Geometry: final body of the model. Coordinates: model frame, mm. A direction names the side the tool comes from. Give positions to 0.01 mm unless a question says otherwise; leave off trailing zeros. Loops run counter-clockwise (first coordinate to the right, second up) from the corner with the lowest first, then second, coordinate; pieces in that order, holes last. Notation, with made-up numbers: (46.25, 23) -> (93.25, 23) arc R23 cw to (93.25, 61) -> close; hole circle Ø6 at (49, -39.5). An arc over 180 degrees is marked (long way). One line per question, with ' | ' between items. Start each with the question number.
Item 1: Mould query, pull axis Y, two halves, no side actions, for faces 6 (the flat face through (0, 12, 11)), 7 (the flat face through (7, 25.725, 11)), 8 (the flat face through (15, -15, 11)). Classes: released by +Y, released by -Y, zero draft, split by the parting line, or undercut.
Item 2: Material intervals for line 1 along Y through (x, z) = (5.5, 11.25) (3 decimals); line 2 along X through (y, z) = (-7.5, 9.5) (3 decimals); line 3 along X through (y, z) = (14.5, 7), sorted ascending. Write a range as [from, to].
Item 3: Pin query (flat end, axial travel): P1, Ø1.5, axis at x = -49, z = 19, coming from the +Y side; P2, Ø6, axis at y = 1.5, z = 19.5, coming from the -X side; P3, Ø4, axis at x = -52, z = 13, coming from the -Y side; P4, Ø6.5, axis at y = -14.5, z = 8.5, coming from the +X side. Return the tip coordinate at first contact, or that it passes through.
Item 4: Section B-B on z = 12.25. Return loops of the section in (x, y) (3 decimals), then the cut area to 3 significant figures.
Item 5: Set-up query: faces 1 (the flat face through (-25, -20, 11)), 2 (the flat face through (7, 19, 17.725)), 3 (the flat face through (-49, -5, 11)), 4 (the flat face through (-51.9, -10, 21.2)), 5 (the flat face through (-11.7, -0.2, 22)). Return all of +Z, -Z, +X, -X, +Y, -Y with unobstructed straight access to the full face (end or side cutting, diameter ignored); none if empty.
Item 6: Section C-C on y = 8.5. Return loops of the section in (x, z), then the cut area to 3 significant figures.
Item 7: Section A-A on x = 1.5. Return loops of the section in (y, z) (3 decimals).
Item 8: Section D-D on x = -20.5. Return loops of the section in (y, z).
from build123d import *

# Parameters (mm, degrees)
PAD_DEPTH       = 22
SKETCH001_W     = 13.45
SKETCH001_H     = 13.45
POCKET_DEPTH    = 15
SKETCH002_W     = 13.45
SKETCH002_H     = 13.45
POCKET001_DEPTH = 15
CHAMFER_SIZE    = 10
POCKET002_DEPTH = 5
CHAMFER001_SIZE = 2


with BuildPart() as part:
    # Sketch → Pad (new body)
    with BuildSketch(Plane.XY):
        Polygon((0, 30), (0, 0), (-60, 0), (-60, -20), (20, -20), (20, 30), align=None)
    extrude(amount=PAD_DEPTH)

    # Sketch001 (on Face1 of Pad) → Pocket (cut)
    with BuildSketch(Plane(origin=(0, 0, 0), x_dir=(0, -1, 0), z_dir=(-1, 0, 0))):
        with Locations((-19, 11)):
            Rectangle(SKETCH001_W, SKETCH001_H)
    extrude(amount=-POCKET_DEPTH, mode=Mode.SUBTRACT)

    # Sketch002 (on Face12 of Pocket) → Pocket001 (cut)
    with BuildSketch(Plane.XZ.offset(20)):
        with Locations((-49, 11)):
            Rectangle(SKETCH002_W, SKETCH002_H)
    extrude(amount=-POCKET001_DEPTH, mode=Mode.SUBTRACT)

    # Chamfer
    chamfer_edges = [part.edges().sort_by_distance(p)[0] for p in [
        (20, -20, 11),
    ]]
    chamfer(chamfer_edges, length=CHAMFER_SIZE)

    # Sketch003 (on Face9 of Chamfer) → Pocket002 (cut)
    with BuildSketch(Plane.XY.offset(22)):
        Polygon((9.295837, 17.3), (10.704163, 17.3), (11.7, 18.295837), (11.7, 19.704163), (10.704163, 20.7), (9.295837, 20.7), (8.3, 19.704163), (8.3, 18.295837), align=None)
        Polygon((-47.3, -10.704163), (-47.3, -9.295837), (-48.295837, -8.3), (-49.704163, -8.3), (-50.7, -9.295837), (-50.7, -10.704163), (-49.704163, -11.7), (-48.295837, -11.7), align=None)
    extrude(amount=-POCKET002_DEPTH, mode=Mode.SUBTRACT)

    # Chamfer001
    chamfer001_edges = [part.edges().sort_by_distance(p)[0] for p in [
        (-50.7, -10, 22),
        (-50.202082, -8.797918, 22),
        (-49, -8.3, 22),
        (-47.797918, -8.797918, 22),
        (-47.3, -10, 22),
        (-47.797918, -11.202082, 22),
        (-49, -11.7, 22),
        (-50.202082, -11.202082, 22),
        (8.3, 19, 22),
        (8.797918, 20.202082, 22),
        (10, 20.7, 22),
        (11.202082, 20.202082, 22),
        (11.7, 19, 22),
        (11.202082, 17.797918, 22),
        (10, 17.3, 22),
        (8.797918, 17.797918, 22),
    ]]
    chamfer(chamfer001_edges, length=CHAMFER001_SIZE)


solid = part.part
Result sheet:
1) face 6: zero draft | face 7: undercut | face 8: released by -Y
2) line 1: y = [-20, 12.275], [25.725, 30] | line 2: x = [-60, -55.725], [-42.275, 20] | line 3: x = [15, 20]
3) P1: stops at y = 0 | P2: stops at x = -60 | P3: stops at y = -5 | P4: stops at x = 18.75
4) outline: (-60, -20) -> (-55.725, -20) -> (-55.725, -5) -> (-42.275, -5) -> (-42.275, -20) -> (10, -20) -> (20, -10) -> (20, 30) -> (0, 30) -> (0, 25.725) -> (15, 25.725) -> (15, 12.275) -> (0, 12.275) -> (0, 0) -> (-60, 0) -> close | area: 1,750 mm²
5) face 1: +Z, -Z, +X, -X, -Y | face 2: -X | face 3: -Y | face 4: +Z | face 5: +Z, +X, -X, +Y, -Y
6) outline: (0, 0) -> (20, 0) -> (20, 22) -> (0, 22) -> close | area: 440 mm²
7) outline: (-20, 0) -> (30, 0) -> (30, 22) -> (-20, 22) -> close; hole (12.275, 4.275) -> (25.725, 4.275) -> (25.725, 17.725) -> (12.275, 17.725) -> close
8) outline: (-20, 0) -> (0, 0) -> (0, 22) -> (-20, 22) -> close
